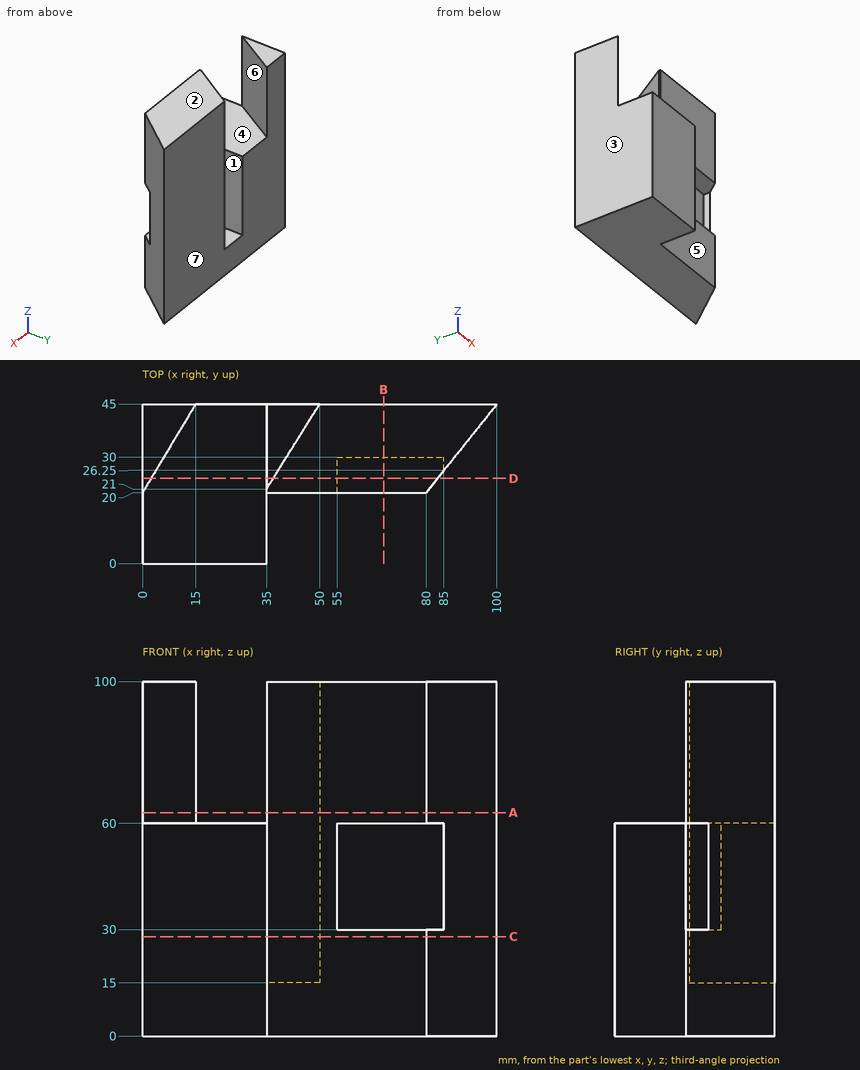
Here's the drawing with two shaded views (mm, measured from the low corner). I have some questions. A direction names the side the tool comes from. Round coordinates to 2 decimals unless told otherwise and drop trailing zeros. Loops run counter-clockwise (first coordinate to the right, second up) from the corner with the lowest first, then second, coordinate; pieces in that order, holes last. Notation, with made-up numbers: M 27.5,43 L 46.5,43 A21 cw 46.5,47 Z; hole C -17,-20 d10. An arc over 180 degrees is marked long. Answer as a JSON object with one key per item and string values. Group by question number.
Q1. Imagine slicing it at C-C, the plane z = 28. Please give me the cut outline in (x, y).
Q2. Imagine slicing it at B-B, the plane x = 68. Please give me the cut outline in (y, z).
Q3. Please list where these lines run through material, in increasing order: L1, parallel to Z at x = 20, y = 19; L2, parallel to Y at x = 56, z = 93.5; L3, parallel to Z at x = 66, y = 21.
Q4. Will these pins go through, and if not, where does the flat tip stop? pin 1 (13.5 mm diameter, centred on x = 66.5, z = 43, fed in from -Y); pin 2 (22 mm diameter, centred on y = 14.5, z = 25, fed in from +X); pin 3 (24 mm diameter, centred on x = 76.5, z = 50.5, fed in from -Y).
Q5. On a 3-axis mill with a long thin cutter (end or side, diameter ignored), from which of +Z, -Z, +X, -X, +Y, -Y can I reach the whole of each face in a straight line? I mean the marked faces 5, 6 and 7. Say none if no direction works.
Q6. Imagine slicing it at D-D, the plane y = 24. Please give me the cut outline in (x, z) (3 decimals).
Q7. Imagine slicing it at A-A, the plane z = 63. Please give me the cut outline in (x, y), then the cut area to 3 significant figures.
Q8. We'd pull the mould along X, two halves only. Please class the marked faces 1, 2, 3 and 4: +X half, -X half, draft (parallel to the pull), parting line (faces both ways), or undercut.
Findings:
{
 "1": {"outline": "M 0,0 L 35,0 L 35,20 L 80,20 L 100,45 L 50,45 L 35,21 L 35,45 L 0,45 Z"},
 "2": {"outline": "M 20,0 L 45,0 L 45,100 L 20,100 L 20,60 L 30,60 L 30,30 L 20,30 Z"},
 "3": {"L1": "z = 0 to 60", "L2": "y = 20 to 45", "L3": "z = 0 to 30, 60 to 100"},
 "4": {"pin 1": "stops at y = 30", "pin 2": "stops at x = 84.4", "pin 3": "stops at y = 20"},
 "5": {"face 5": "+Z, -Z, +X, -Y", "face 6": "+Z, -Y", "face 7": "+Z, -Z, +X, -X, +Y"},
 "6": {"outline": "M 0,0 L 83.2,0 L 83.2,30 L 55,30 L 55,60 L 83.2,60 L 83.2,100 L 36.875,100 L 36.875,15 L 35,15 L 35,60 L 2.4,60 L 2.4,100 L 0,100 Z"},
 "7": {"outline": "M 0,20 L 15,45 L 0,45 Z; M 35,20 L 80,20 L 100,45 L 50,45 L 35,21 Z", "area": "1,380 mm2"},
 "8": {"face 1": "undercut", "face 2": "draft", "face 3": "-X half", "face 4": "undercut"}
}
